from build123d import *

# Parameters (mm, degrees)
SKETCH1_W           = 5.08
SKETCH1_H           = 5.08
BOSS_EXTRUDE1_DEPTH = 1.44
SKETCH2_R           = 1.5
BOSS_EXTRUDE2_DEPTH = 10
SKETCH3_R           = 1.75
BOSS_EXTRUDE3_DEPTH = 2.5
CHAMFER1_SIZE       = 0.3


with BuildPart() as part:
    # Sketch1 → Boss-Extrude1 (new body)
    with BuildSketch(Plane(origin=(0, 0, 0), x_dir=(1, 0, 0), z_dir=(0, 1, 0))):
        Rectangle(SKETCH1_W, SKETCH1_H)
    extrude(amount=BOSS_EXTRUDE1_DEPTH)

    # Sketch2 → Boss-Extrude2 (add)
    with BuildSketch(Plane.XZ.offset(-1.44)):
        with Locations(Location((0, 0, 0), (0, 0, 90))):
            Circle(SKETCH2_R)
    extrude(amount=BOSS_EXTRUDE2_DEPTH)

    # Sketch3 → Boss-Extrude3 (add)
    with BuildSketch(Plane(origin=(0, 1.44, 0), x_dir=(1, 0, 0), z_dir=(0, 1, 0))):
        with Locations(Location((0, 0, 0), (0, 0, 270))):
            Circle(SKETCH3_R)
    extrude(amount=BOSS_EXTRUDE3_DEPTH)

    # Chamfer1
    chamfer1_edges = [part.edges().sort_by_distance(p)[0] for p in [
        (2.54, 1.44, 0),
        (-2.54, 1.44, 0),
        (2.54, 0, 0),
        (-2.54, 0, 0),
    ]]
    chamfer(chamfer1_edges, length=CHAMFER1_SIZE)


solid = part.part
Geometry: final body of the model. Coordinates: model frame, mm. A direction names the side the tool comes from. Round coordinates to 2 decimals unless told otherwise and drop trailing zeros. Order: outer loops, then holes, each group sorted by start corner. A loop starts at its lowest first (then second) coordinate and runs counter-clockwise, first axis right, second up.
Q1. Section C-C, the plane y = -2.75. Output: boundary loops of the cut face in (x, z).
Result sheet:
outline: circle Ø3 at (0, 0)
Q2. Pin query (flat end, axial travel): pin 1 (1 mm diameter, centred on y = -5, z = -0.5, fed in from +X). Return the tip coordinate at first contact, or that it passes through.
Result sheet:
pin 1: stops at x = 1.5
Q3. Material intervals for probe 1 along Y at (x, z) = (1.65, -1.1); probe 2 along Z at (x, y) = (-0.1, 2); probe 3 along Z at (x, y) = (0.9, 3.25), sorted ascending.
Result sheet:
probe 1: y = 0 to 1.44
probe 2: z = -1.75 to 1.75
probe 3: z = -1.5 to 1.5
Q4. Access query for faces 1 (the face through (-0.45, -4.22, 1.43)), 2 (the face through (0, 1, -2.54)), 3 (the face through (-1.71, 2.67, -0.38)). Directions: +Z, -Z, +X, -X, +Y, -Y. A direction counts if a zero-diameter tool reaches every point of the face in a straight line with its end or side. Return the directions, or none.
Result sheet:
face 1: -Y
face 2: -Z, +X, -X, +Y, -Y
face 3: +Y
Q5. Section D-D, the plane z = -2.05. Output: boundary loops of the cut face in (x, y).
Result sheet:
outline: (-2.54, 0.3) - (-2.24, 0) - (2.24, 0) - (2.54, 0.3) - (2.54, 1.14) - (2.24, 1.44) - (-2.24, 1.44) - (-2.54, 1.14) - close
Q6. Section B-B, the plane z = 0. Output: boundary loops of the cut face in (x, y).
Result sheet:
outline: (-2.54, 0.3) - (-2.24, 0) - (-1.5, 0) - (-1.5, -8.56) - (1.5, -8.56) - (1.5, 0) - (2.24, 0) - (2.54, 0.3) - (2.54, 1.14) - (2.24, 1.44) - (1.75, 1.44) - (1.75, 3.94) - (-1.75, 3.94) - (-1.75, 1.44) - (-2.24, 1.44) - (-2.54, 1.14) - close
Q7. Section A-A, the plane x = 0. Output: boundary loops of the cut face in (y, z).
Result sheet:
outline: (-8.56, -1.5) - (0, -1.5) - (0, -2.54) - (1.44, -2.54) - (1.44, -1.75) - (3.94, -1.75) - (3.94, 1.75) - (1.44, 1.75) - (1.44, 2.54) - (0, 2.54) - (0, 1.5) - (-8.56, 1.5) - close
